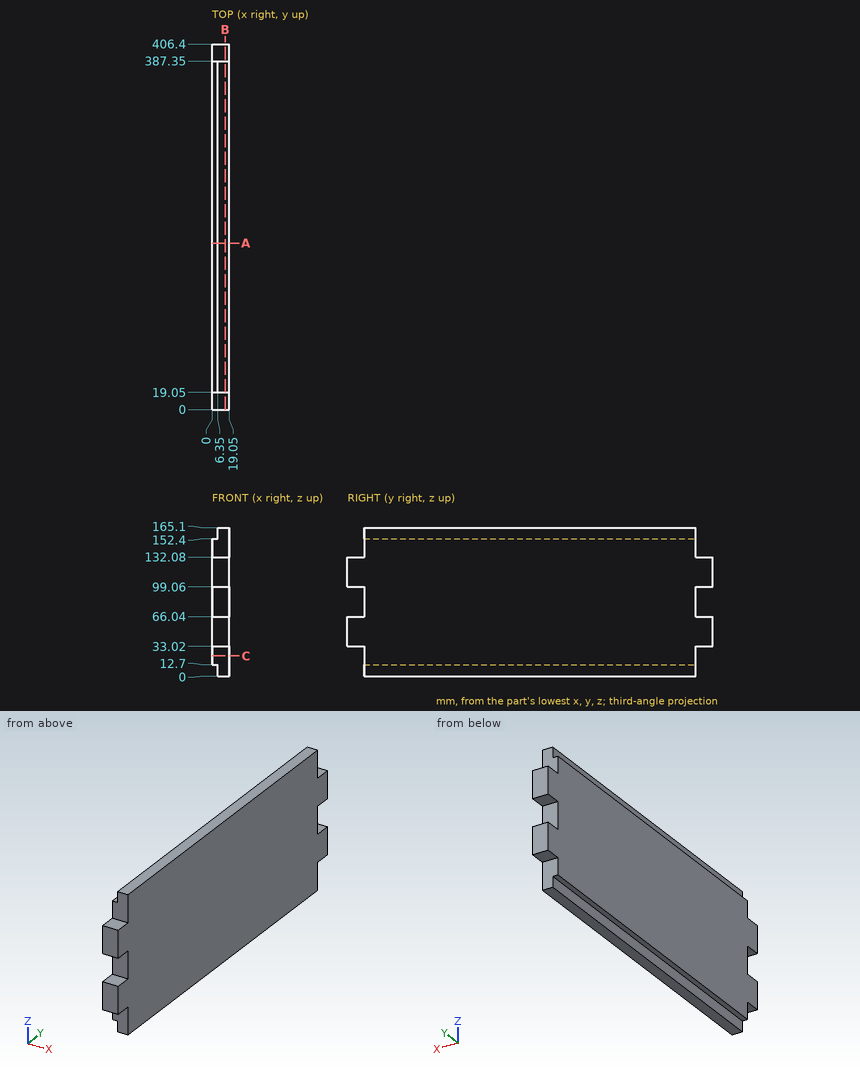
Could you check a few things on this drawing? It's one solid part, dimensions in mm from its lowest x, y, z. Coordinates: 2 decimals unless noted, no trailing zeros. Order: outer loops, then holes, each group sorted by start corner. A loop starts at its lowest first (then second) coordinate and runs counter-clockwise, first axis right, second up. Notation, with made-up numbers: (58, 65) - (107, 65) arc R34 ccw to (107, 98) - close; hole circle Ø2 at (18.25, 51). An arc over 180 degrees is marked (long way). One line per question, with ' | ' between items. Start each with the question number.
1. I'm going to push flat-ended pins straight in: pin 1 Ø1 at (x, z) = (17, 17.5) entering from -Y; pin 2 Ø5.5 at (x, z) = (9, 18.5) entering from +Y; pin 3 Ø5.5 at (x, y) = (13.5, 10) entering from -Z; pin 4 Ø4 at (y, z) = (116.5, 140.5) entering from -X. Where does each tip first touch, or does it pass through?
2. Please list where these lines run through material, in increasing order: line 1 along Y through (x, z) = (14, 18); line 2 along Z through (x, y) = (2.75, 353). Write a range as [from, to].
3. If we section it at C-C (z = 22.5): Write out the boundary of the cut face in (x, y), and give its area (3 significant figures).
4. If we section it at A-A (y = 185): Write out the boundary of the cut face in (x, z).
5. If we section it at B-B (x = 14.5): Write out the boundary of the cut face in (y, z).
Model answer:
1) pin 1: stops at y = 19.05 | pin 2: stops at y = 387.35 | pin 3: stops at z = 33.02 | pin 4: stops at x = 0
2) line 1: y = [19.05, 387.35] | line 2: z = [12.7, 152.4]
3) outline: (0, 19.05) - (19.05, 19.05) - (19.05, 387.35) - (0, 387.35) - close | area: 7,020 mm²
4) outline: (0, 12.7) - (6.35, 12.7) - (6.35, 0) - (19.05, 0) - (19.05, 165.1) - (6.35, 165.1) - (6.35, 152.4) - (0, 152.4) - close
5) outline: (0, 33.02) - (19.05, 33.02) - (19.05, 0) - (387.35, 0) - (387.35, 33.02) - (406.4, 33.02) - (406.4, 66.04) - (387.35, 66.04) - (387.35, 99.06) - (406.4, 99.06) - (406.4, 132.08) - (387.35, 132.08) - (387.35, 165.1) - (19.05, 165.1) - (19.05, 132.08) - (0, 132.08) - (0, 99.06) - (19.05, 99.06) - (19.05, 66.04) - (0, 66.04) - close
